For this review, use the dimensioned drawing (mm, ordinates from the lowest corner) and the shaded views. A direction names the side the tool comes from. Round coordinates to 2 decimals unless told otherwise and drop trailing zeros. Loops run counter-clockwise (first coordinate to the right, second up) from the corner with the lowest first, then second, coordinate; pieces in that order, holes last. Notation, with made-up numbers: M 70,-27.75 L 95,-27.75 A12 ccw 95,-11.75 Z; hole C 34.25,60.25 d9. An arc over 180 degrees is marked long. One line per item, written item: value. Start each with the question number.
Item 1: Mouldability with a two-part tool opening along X and no side actions: class the marked faces 5, 6 and 7 as released by +X, released by -X, zero draft, split by the parting line, or undercut.
Item 2: We need section B-B (y = 24). Write out the cut boundary in (x, z), then the cut area to 3 significant figures.
Item 3: For the marked faces 1, 2, 3 and 4, list the 3-axis set-ups (+Z, -Z, +X, -X, +Y, -Y) from which the entire face can be reached by the end or side of a thin tool; tool diameter is ignored.
Item 4: We need section A-A (z = 10). Write out the cut boundary in (x, y).
Item 5: We need section D-D (y = 51). Write out the cut boundary in (x, z), then the cut area to 3 significant figures.
Item 6: Clearance check with flat-ended pins moving along their axes: pin 1 (4 mm diameter, centred on y = 24, z = 9, fed in from +X); pin 2 (7.5 mm diameter, centred on y = 32.5, z = 4.5, fed in from -X); pin 3 (1 mm diameter, centred on x = 25, y = 9, fed in from -Z) (3 decimals); pin 4 (5 mm diameter, centred on x = 28, z = 7.5, fed in from +Y). State where each tip first meets the part, or that it passes through.
Item 7: For line 1 along X through (y, z) = (47, 9); line 2 along Z through (x, y) = (28, 52); line 3 along Z through (x, y) = (9.5, 28), list the stretches that pass through material, from the lowest coordinate up.
Item 8: We need section C-C (x = 4.5). Write out the cut boundary in (y, z), then the cut area to 3 significant figures.
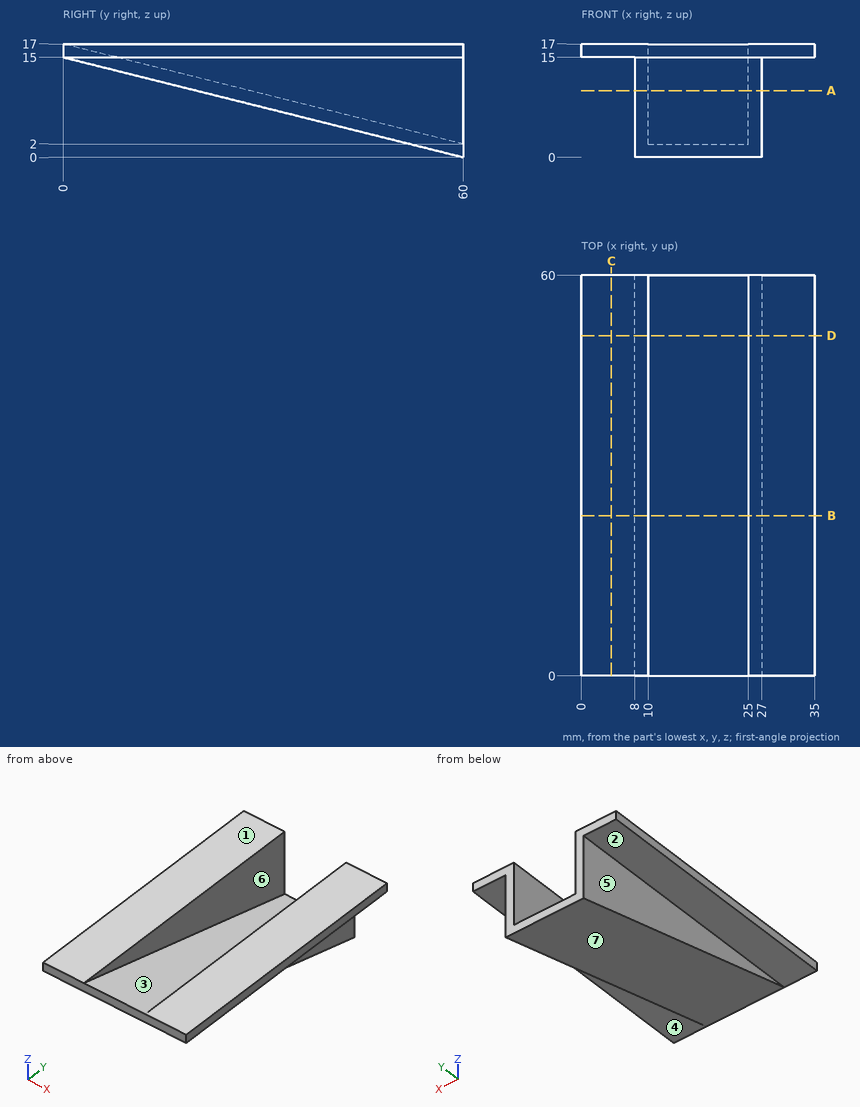
A:
1. face 5: released by -X
1. face 6: undercut
1. face 7: zero draft
2. outline: M 0,15 L 8,15 L 8,9 L 27,9 L 27,15 L 35,15 L 35,17 L 25,17 L 25,11 L 10,11 L 10,17 L 0,17 Z
2. area: 94.0 mm2
3. face 1: +Z, +X, -X, +Y, -Y
3. face 2: -Z, -X, +Y, -Y
3. face 3: +Z, +Y
3. face 4: -Z, +X, +Y, -Y
4. outline: M 8,20 L 27,20 L 27,60 L 25,60 L 25,28 L 10,28 L 10,60 L 8,60 Z
5. outline: M 0,15 L 8,15 L 8,2.25 L 27,2.25 L 27,15 L 35,15 L 35,17 L 25,17 L 25,4.25 L 10,4.25 L 10,17 L 0,17 Z
5. area: 121 mm2
6. pin 1: x = 27
6. pin 2: x = 8
6. pin 3: z = 12.625
6. pin 4: y = 60
7. line 1: 8 to 10, 25 to 27
7. line 2: 15 to 17
7. line 3: 8 to 17
8. outline: M 0,15 L 60,15 L 60,17 L 0,17 Z
8. area: 120 mm2
